from build123d import *

# Parameters (mm, degrees)
SM_BASE_FLANGE_1_OUTLINE_R   = 2.1
SM_BASE_FLANGE_1_OUTLINE_R_2 = 1.6
SM_BASE_FLANGE_1_OUTLINE_R_3 = 8.4
SM_BASE_FLANGE_1_DEPTH       = 1.5
SKETCH_2_R                   = 1.6
CUT_EXTRUDE_1_DEPTH          = 10
SKETCH_4_R                   = 2.1
CUT_EXTRUDE_2_DEPTH          = 1.5
SKETCH_6_R                   = 1.6
CUT_EXTRUDE_4_DEPTH          = 1.5


# Read off the part's stored shape, not the designer's step: 基体-法兰1
with BuildPart() as part:
    # 基体-法兰1 outline → 基体-法兰1 (new body)
    with BuildSketch(Plane.XY):
        with BuildLine():
            ThreePointArc((-145, -38.405728739), (0, -150), (145, -38.405728739))
            Line((145, -38.405728739), (145, 38.405728739))
            ThreePointArc((145, 38.405728739), (0, 150), (-145, 38.405728739))
            Line((-145, 38.405728739), (-145, -38.405728739))
        make_face()
        with Locations((-78.675798494, -112.770480318)):
            Circle(SM_BASE_FLANGE_1_OUTLINE_R, mode=Mode.SUBTRACT)
        with Locations((-112.770480318, -78.675798494)):
            Circle(SM_BASE_FLANGE_1_OUTLINE_R, mode=Mode.SUBTRACT)
        with Locations((-58.324201506, -124.520480318)):
            Circle(SM_BASE_FLANGE_1_OUTLINE_R, mode=Mode.SUBTRACT)
        with Locations((-11.75, -137)):
            Circle(SM_BASE_FLANGE_1_OUTLINE_R, mode=Mode.SUBTRACT)
        with Locations((-25, -115)):
            Circle(SM_BASE_FLANGE_1_OUTLINE_R, mode=Mode.SUBTRACT)
        with Locations((-124.520480318, -58.324201506)):
            Circle(SM_BASE_FLANGE_1_OUTLINE_R, mode=Mode.SUBTRACT)
        with Locations((-79, -49.959487412)):
            Circle(SM_BASE_FLANGE_1_OUTLINE_R, mode=Mode.SUBTRACT)
        with Locations((-137, -11.75)):
            Circle(SM_BASE_FLANGE_1_OUTLINE_R, mode=Mode.SUBTRACT)
        with Locations((-83, -25)):
            Circle(SM_BASE_FLANGE_1_OUTLINE_R, mode=Mode.SUBTRACT)
        with Locations((-30.75, -4.524131076)):
            Circle(SM_BASE_FLANGE_1_OUTLINE_R_2, mode=Mode.SUBTRACT)
        with Locations((11.75, -137)):
            Circle(SM_BASE_FLANGE_1_OUTLINE_R, mode=Mode.SUBTRACT)
        with Locations((25, -115)):
            Circle(SM_BASE_FLANGE_1_OUTLINE_R, mode=Mode.SUBTRACT)
        with Locations((58.324201506, -124.520480318)):
            Circle(SM_BASE_FLANGE_1_OUTLINE_R, mode=Mode.SUBTRACT)
        with BuildLine():
            Line((40, -102.5), (-40, -102.5))
            ThreePointArc((-40, -102.5), (-47.5, -95), (-40, -87.5))
            Line((-40, -87.5), (40, -87.5))
            ThreePointArc((40, -87.5), (47.5, -95), (40, -102.5))
        make_face(mode=Mode.SUBTRACT)
        with Locations((78.675798494, -112.770480318)):
            Circle(SM_BASE_FLANGE_1_OUTLINE_R, mode=Mode.SUBTRACT)
        with Locations((112.770480318, -78.675798494)):
            Circle(SM_BASE_FLANGE_1_OUTLINE_R, mode=Mode.SUBTRACT)
        with Locations((30.75, -4.524131076)):
            Circle(SM_BASE_FLANGE_1_OUTLINE_R_2, mode=Mode.SUBTRACT)
        with Locations((79, -72.959487412)):
            Circle(SM_BASE_FLANGE_1_OUTLINE_R, mode=Mode.SUBTRACT)
        with Locations((124.520480318, -58.324201506)):
            Circle(SM_BASE_FLANGE_1_OUTLINE_R, mode=Mode.SUBTRACT)
        with Locations((137, -11.75)):
            Circle(SM_BASE_FLANGE_1_OUTLINE_R, mode=Mode.SUBTRACT)
        with Locations((-137, 11.75)):
            Circle(SM_BASE_FLANGE_1_OUTLINE_R, mode=Mode.SUBTRACT)
        with BuildLine():
            Line((-112.567715637, -50.975868924), (-112.567715637, 50.975868924))
            ThreePointArc((-112.567715637, 50.975868924), (-105.067715637, 58.475868924), (-97.567715637, 50.975868924))
            Line((-97.567715637, 50.975868924), (-97.567715637, -50.975868924))
            ThreePointArc((-97.567715637, -50.975868924), (-105.067715637, -58.475868924), (-112.567715637, -50.975868924))
        make_face(mode=Mode.SUBTRACT)
        with Locations((-83, 35)):
            Circle(SM_BASE_FLANGE_1_OUTLINE_R, mode=Mode.SUBTRACT)
        with Locations((-124.520480318, 58.324201506)):
            Circle(SM_BASE_FLANGE_1_OUTLINE_R, mode=Mode.SUBTRACT)
        with Locations((-30.75, 71.975868924)):
            Circle(SM_BASE_FLANGE_1_OUTLINE_R_2, mode=Mode.SUBTRACT)
        with Locations((-112.770480318, 78.675798494)):
            Circle(SM_BASE_FLANGE_1_OUTLINE_R, mode=Mode.SUBTRACT)
        with Locations((-79, 82.040512588)):
            Circle(SM_BASE_FLANGE_1_OUTLINE_R, mode=Mode.SUBTRACT)
        with Locations((-78.675798494, 112.770480318)):
            Circle(SM_BASE_FLANGE_1_OUTLINE_R, mode=Mode.SUBTRACT)
        with Locations((-58.324201506, 124.520480318)):
            Circle(SM_BASE_FLANGE_1_OUTLINE_R, mode=Mode.SUBTRACT)
        with Locations((-11.75, 137)):
            Circle(SM_BASE_FLANGE_1_OUTLINE_R, mode=Mode.SUBTRACT)
        Circle(SM_BASE_FLANGE_1_OUTLINE_R_3, mode=Mode.SUBTRACT)
        with Locations((30.75, 71.975868924)):
            Circle(SM_BASE_FLANGE_1_OUTLINE_R_2, mode=Mode.SUBTRACT)
        with BuildLine():
            Line((86.5, -50.975868924), (86.5, 50.975868924))
            ThreePointArc((86.5, 50.975868924), (94, 58.475868924), (101.5, 50.975868924))
            Line((101.5, 50.975868924), (101.5, -50.975868924))
            ThreePointArc((101.5, -50.975868924), (94, -58.475868924), (86.5, -50.975868924))
        make_face(mode=Mode.SUBTRACT)
        with Locations((137, 11.75)):
            Circle(SM_BASE_FLANGE_1_OUTLINE_R, mode=Mode.SUBTRACT)
        with Locations((124.520480318, 58.324201506)):
            Circle(SM_BASE_FLANGE_1_OUTLINE_R, mode=Mode.SUBTRACT)
        with BuildLine():
            Line((40, 92.5), (-40, 92.5))
            ThreePointArc((-40, 92.5), (-47.5, 100), (-40, 107.5))
            Line((-40, 107.5), (40, 107.5))
            ThreePointArc((40, 107.5), (47.5, 100), (40, 92.5))
        make_face(mode=Mode.SUBTRACT)
        with Locations((11.75, 137)):
            Circle(SM_BASE_FLANGE_1_OUTLINE_R, mode=Mode.SUBTRACT)
        with Locations((58.324201506, 124.520480318)):
            Circle(SM_BASE_FLANGE_1_OUTLINE_R, mode=Mode.SUBTRACT)
        with Locations((79, 82.040512588)):
            Circle(SM_BASE_FLANGE_1_OUTLINE_R, mode=Mode.SUBTRACT)
        with Locations((112.770480318, 78.675798494)):
            Circle(SM_BASE_FLANGE_1_OUTLINE_R, mode=Mode.SUBTRACT)
        with Locations((78.675798494, 112.770480318)):
            Circle(SM_BASE_FLANGE_1_OUTLINE_R, mode=Mode.SUBTRACT)
    extrude(amount=SM_BASE_FLANGE_1_DEPTH)

    # 草图2 → 切除-拉伸1 (cut)
    with BuildSketch(Plane.XY.offset(1.5)):
        with Locations((40, -34)):
            Circle(SKETCH_2_R)
        with Locations((40, 31)):
            Circle(SKETCH_2_R)
        with Locations((21.043, -13.55)):
            Circle(SKETCH_2_R)
        with Locations((-39, -27)):
            Circle(SKETCH_2_R)
        with Locations((-29.75, 29.67)):
            Circle(SKETCH_2_R)
        with Locations((21.043, 14.45)):
            Circle(SKETCH_2_R)
    extrude(amount=-CUT_EXTRUDE_1_DEPTH, mode=Mode.SUBTRACT)

    # 草图4 → 切除-拉伸2 (cut)
    with BuildSketch(Plane(origin=(0, 0, 0), x_dir=(-1, 0, 0), z_dir=(0, 0, -1))):
        with Locations((-60, 110)):
            Circle(SKETCH_4_R)
        with Locations((60, 110)):
            Circle(SKETCH_4_R)
    extrude(amount=-CUT_EXTRUDE_2_DEPTH, mode=Mode.SUBTRACT)

    # 草图6 → 切除-拉伸4 (cut)
    with BuildSketch(Plane.XY.offset(1.5)):
        with Locations((42.500000131, 41)):
            Circle(SKETCH_6_R)
        with Locations((42.500001181, -31.28)):
            Circle(SKETCH_6_R)
        with Locations((-43.299998782, -33.8)):
            Circle(SKETCH_6_R)
        with Locations((-43.299999908, 43.65)):
            Circle(SKETCH_6_R)
    extrude(amount=-CUT_EXTRUDE_4_DEPTH, mode=Mode.SUBTRACT)


solid = part.part
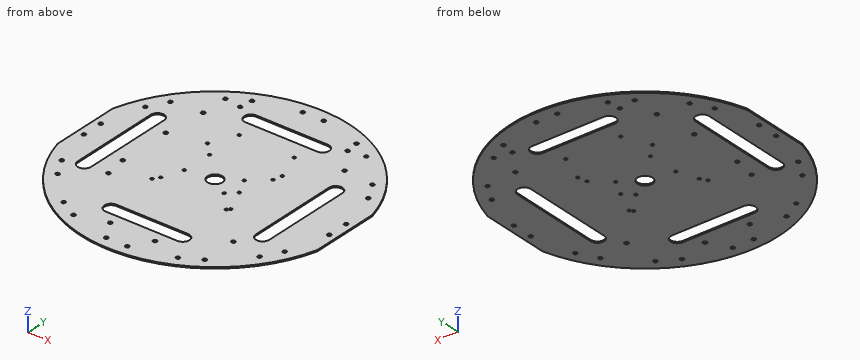
Geometry check sheet. Reference: the model listing, model coordinates, mm. Give positions to 0.01 mm unless a question says otherwise; leave off trailing zeros. Order: outer loops, then holes, each group sorted by start corner. A loop starts at its lowest first (then second) coordinate and runs counter-clockwise, first axis right, second up. Notation, with made-up numbers: M 54,3.25 L 59,3.25 A20 ccw 59,13.25 Z; hole C 83,-23.75 d10. An arc over 180 degrees is marked long. Use a Markdown table: item, result.
Item 1: Material ranges on line 1 along X through (y, z) = (79, 1.4); line 2 along Y through (x, z) = (-32.5, 0.95); line 3 along X through (y, z) = (-112.5, 0.45), recorded low to high.
Answers follow:
| item | result |
|---|---|
| line 1 | x = -127.51 to -114.85, -110.7 to 110.7, 114.85 to 127.51 |
| line 2 | y = -146.44 to -102.5, -87.5 to 92.5, 107.5 to 146.44 |
| line 3 | x = -99.22 to -80.76, -76.59 to 76.59, 80.76 to 99.22 |
Item 2: Section check C-C (x = -71). Record the cut outline in (y, z), and give its area (3 significant figures).
Answers follow:
| item | result |
|---|---|
| outline | M -132.13,0 L 132.13,0 L 132.13,1.5 L -132.13,1.5 Z |
| area | 396 mm2 |
Item 3: Section check B-B (x = 107). Record the cut outline in (y, z).
Answers follow:
| item | result |
|---|---|
| outline | M -105.12,0 L 105.12,0 L 105.12,1.5 L -105.12,1.5 Z |
Item 4: Section check A-A (z = 0.9). State how many separate pieces and enclosed holes the cut face has, and give its area (3 significant figures).
Answers follow:
| item | result |
|---|---|
| separate pieces | 1 |
| enclosed holes | 53 |
| area | 63,200 mm2 |
Item 5: Depth check by flat-ended pin: P1, Ø5.5, axis at x = -58.32, y = 124.52, coming from the -Z side; P2, Ø2.5, axis at x = 137, y = -11.75, coming from the +Z side. Enter the tip coordinate at first touch or a pass-through.
Answers follow:
| item | result |
|---|---|
| P1 | stops at z = 0 |
| P2 | passes through |
